Geometry: final body of the model. Coordinates: model frame, mm. A direction names the side the tool comes from. Coordinates: 2 decimals unless noted, no trailing zeros. Loops run counter-clockwise (first coordinate to the right, second up) from the corner with the lowest first, then second, coordinate; pieces in that order, holes last. Notation, with made-up numbers: M -37,74 L -32,74 A32 ccw -32,113 Z; hole C 37,50.25 d5. An arc over 180 degrees is marked long. Write item = value, one per line. Start each with the question number.
```python
from build123d import *

# Parameters (mm, degrees)
BOSS_EXTRUDE1_DEPTH = 10
SKETCH2_W           = 1.8
SKETCH2_H           = 8
BOSS_EXTRUDE2_DEPTH = 3


with BuildPart() as part:
    # Sketch1 → Boss-Extrude1 (new body)
    with BuildSketch(Plane(origin=(0, 0, 0), x_dir=(1, 0, 0), z_dir=(0, 1, 0))):
        Polygon((0, 0), (7.2, 0), (7.2, -6), (10.2, -6), (11, 3), (0, 3), align=None)
    extrude(amount=BOSS_EXTRUDE1_DEPTH)

    # Sketch2 → Boss-Extrude2 (add)
    with BuildSketch(Plane.XY):
        with Locations((2.5, 5)):
            Rectangle(SKETCH2_W, SKETCH2_H)
    extrude(amount=BOSS_EXTRUDE2_DEPTH)


solid = part.part
```
Item 1: Reachability of faces 4 (the flat face through (3.4, 5, 1)), 5 (the flat face through (2, 5, 3)), 6 (the flat face through (2, 9, 1)), 7 (the flat face through (7, 0, -1)) from +Z, -Z, +X, -X, +Y, -Y: full face, straight path, thin tool, end or side. Return the list, or none.
Item 2: Pull-direction query (X, two-part tool) for faces 1 (the flat face through (2, 1, 1)), 2 (the flat face through (4, 5, 0)), 3 (the flat face through (0, 5, -2)); classes: released by +X, released by -X, zero draft, split by the parting line, or undercut.
Item 3: Section query A-A (z = 2.75). Return the cut outline in (x, y).
Item 4: Section query C-C (x = 1.75). Return the cut outline in (y, z), plus the area to 3 significant figures.
Item 5: Section query D-D (z = 1.25). Return the cut outline in (x, y).
Item 6: Line query: line 1 (Z direction, x = 5.5, y = 1); line 2 (X direction, y = 7, z = 1); line 3 (Y direction, x = 2, z = 0.5). Output: solid intervals per line, ascending. Write a range as from..to.
Item 7: Section query B-B (y = 9.25). Return the cut outline in (x, z), plus the area to 3 significant figures.
Item 8: First-contact query: pin 1 (2 mm diameter, centred on y = 3, z = 3.5, fed in from +X); pin 2 (6 mm diameter, centred on x = 2, y = 3, fed in from +Z); pin 3 (5 mm diameter, centred on y = 7, z = 2, fed in from -X); pin 4 (0.9 mm diameter, centred on y = 4, z = 1, fed in from -X). Flat tips, straight axial feed; report the tip coordinate or a pass-through.
Verdict:
q1.face_4 = +Z, +Y, -Y
q1.face_5 = +Z, -X, +Y, -Y
q1.face_6 = +Z, -X, +Y
q1.face_7 = +Z, -Z, +X, -X, -Y
q2.face_1 = zero draft
q2.face_2 = undercut
q2.face_3 = released by -X
q3.outline = M 1.6,1 L 3.4,1 L 3.4,9 L 1.6,9 Z; M 7.2,0 L 10.49,0 L 10.49,10 L 7.2,10 Z
q4.outline = M 0,-3 L 10,-3 L 10,0 L 9,0 L 9,3 L 1,3 L 1,0 L 0,0 Z
q4.area = 54.0 mm2
q5.outline = M 1.6,1 L 3.4,1 L 3.4,9 L 1.6,9 Z; M 7.2,0 L 10.62,0 L 10.62,10 L 7.2,10 Z
q6.line_1 = -3..0
q6.line_2 = 1.6..3.4, 7.2..10.64
q6.line_3 = 1..9
q7.outline = M 0,-3 L 11,-3 L 10.2,6 L 7.2,6 L 7.2,0 L 0,0 Z
q7.area = 52.2 mm2
q8.pin_1 = 10.51
q8.pin_2 = 3
q8.pin_3 = 0
q8.pin_4 = 1.6
